from build123d import *

# Parameters (mm, degrees)
PAD_DEPTH = 18


with BuildPart() as part:
    # Sketch → Pad (new body)
    with BuildSketch(Plane.XY):
        Polygon((0, 67), (30, 67), (30, 55), (90, 55), (135.301157, 62.987816), (137.037638, 53.139739), (148.855331, 55.223517), (156.669499, 10.907168), (144.851806, 8.82339), (146.407608, 0), (0, 0), align=None)
    pad = extrude(amount=PAD_DEPTH)

    # Mirrored: Pad across Sketch V_Axis
    add(pad.mirror(Plane(origin=(0, 0, 0), x_dir=(0, 0, 1), z_dir=(1, 0, 0))))


solid = part.part
The model under review builds one solid part; all positions refer to its coordinate system, in mm. A direction names the side the tool comes from. Round coordinates to 2 decimals unless told otherwise and drop trailing zeros. Order: outer loops, then holes, each group sorted by start corner. A loop starts at its lowest first (then second) coordinate and runs counter-clockwise, first axis right, second up. Notation, with made-up numbers: (-12, 41.25) -> (47, 41.25) arc R37 ccw to (47, 79.25) -> close; hole circle Ø10 at (26, 73). An arc over 180 degrees is marked (long way). Use CSV: the item, a comma, the result in double quotes. Start each with the question number.
(1) Consider section A-A on z = 14.75. Write out the cut boundary in (x, y), and give its area (3 significant figures).
(2) Wall thickness on probe 1 along Y at (x, z) = (-71.5, 12.25); probe 2 along X at (y, z) = (40, 12.5); probe 3 along X at (y, z) = (48.5, 8): over which ranges is each line inside the solid? List them lowest first. Write a range as from..to.
(3) Consider section B-B on x = -69.5. Write out the cut boundary in (y, z).
(4) Tool access review of faces 4 (the face through (-145.62, 4.47, 8.87)), 5 (the face through (145.62, 4.47, 8.87)), 6 (the face through (30, 61, 9)), 7 (the face through (-2, 0, 9)): name each direction out of +Z, -Z, +X, -X, +Y, -Y from which nothing blocks a thin tool from reaching the whole face with its end or side.
(5) Insertion check: pin 1 (3 mm diameter, centred on y = 41.5, z = 13.5, fed in from +X); pin 2 (3.5 mm diameter, centred on y = 60.5, z = 10, fed in from -X); pin 3 (3.5 mm diameter, centred on y = 58.5, z = 6, fed in from +X). Each pin has a flat end and moves straight along its axis. Give the tip position at first contact, or say it passes through.
(6) Mouldability with a two-part tool opening along X and no side actions: class faces 1 (the face through (142.864, 54.167, 8.874)), 2 (the face through (-2, 27, 18)), 3 (the face through (152.708, 33.376, 8.874)) as pulls with the +X half, pulls with the -X half, needs draft (parallel to the pull), parting line crosses it, or undercut.
(7) Consider section C-C on y = 49. Write out the cut boundary in (x, z).
Responses:
1,outline,"(-156.67, 10.91) -> (-144.85, 8.82) -> (-146.41, 0) -> (146.41, 0) -> (144.85, 8.82) -> (156.67, 10.91) -> (148.86, 55.22) -> (137.04, 53.14) -> (135.3, 62.99) -> (90, 55) -> (30, 55) -> (30, 67) -> (-30, 67) -> (-30, 55) -> (-90, 55) -> (-135.3, 62.99) -> (-137.04, 53.14) -> (-148.86, 55.22) -> close"
1,area,"17,700 mm²"
2,probe 1,"0..55"
2,probe 2,"-151.54..151.54"
2,probe 3,"-150.04..150.04"
3,outline,"(0, 0) -> (55, 0) -> (55, 18) -> (0, 18) -> close"
4,face 4,"+Z, -Z, -X"
4,face 5,"+Z, -Z, +X"
4,face 6,"+Z, -Z, +Y"
4,face 7,"+Z, -Z, +X, -X, -Y"
5,pin 1,"x = 151.54"
5,pin 2,"x = -136.05"
5,pin 3,"x = 136.4"
6,face 1,"undercut"
6,face 2,"needs draft"
6,face 3,"pulls with the +X half"
7,outline,"(-149.95, 0) -> (149.95, 0) -> (149.95, 18) -> (-149.95, 18) -> close"
